Study the drawing (mm; zero at the part's minimum x, y, z) and answer. Coordinates: 2 decimals unless noted, no trailing zeros. Loops run counter-clockwise (first coordinate to the right, second up) from the corner with the lowest first, then second, coordinate; pieces in that order, holes last. Notation, with made-up numbers: (-21.5, 82) -> (0.5, 82) arc R27 cw to (0.5, 121) -> close; hole circle Ø2 at (-11, -26.75). An arc over 180 degrees is marked (long way). One line per question, with ' | ' between items.
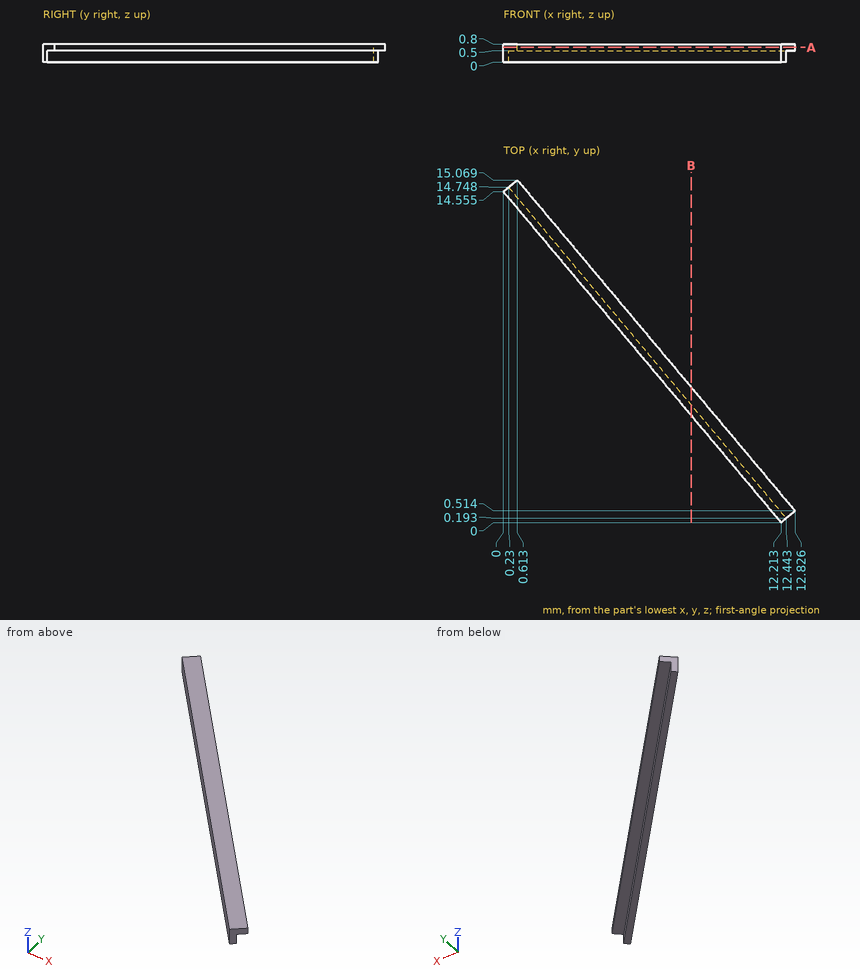
1) Find section A-A (z = 0.65). Write down the section's boundary in (x, y) (1 decimal), plus the area to 3 significant figures.
Check values:
outline: (0, 14.6) -> (12.2, 0) -> (12.8, 0.5) -> (0.6, 15.1) -> close | area: 15.2 mm^2
2) Find section B-B (x = 8.25). Write down the section's boundary in (y, z).
Check values:
outline: (4.72, 0) -> (5.19, 0) -> (5.19, 0.5) -> (5.97, 0.5) -> (5.97, 0.8) -> (4.72, 0.8) -> close
3) Find the intervals of material crossed by line 1 along Z through (x, y) = (4.5, 10); line 2 along X through (y, z) = (7.5, 0.2); line 3 along X through (y, z) = (11, 0.6), in increasing order.
Check values:
line 1: z = 0.5 to 0.8 | line 2: x = 5.92 to 6.31 | line 3: x = 2.98 to 4.03
